Geometry: see drawing. Coordinates: mm, zero at the bounding-box minimum. A direction names the side the tool comes from. Give positions to 0.01 mm unless a question says otherwise; leave off trailing zeros. Write each loop counter-clockwise with the first axis right and the second up, starting at its lowest first coordinate (ties: lowest second). Pieces come first, ordered by that corner, then holes. Notation, with made-up numbers: (6, 65) - (22, 65) arc R25 ccw to (22, 79) - close; hole circle Ø3 at (-11, 9.5). An arc over 180 degrees is marked (long way). One line per question, with ' | ' between items. Start each with the question number.
(1) Ray query, line 1 (Y direction, x = 38, z = 48); line 2 (Y direction, x = 4, z = 13.5); line 3 (X direction, y = 17.5, z = 32). Return the intervals inside material, ascending. Write a range as [from, to].
(2) Section D-D, the plane y = 2. Return loops of the section in (x, z), plus the area to 3 significant figures.
(3) Section B-B, the plane x = 7.5. Return loops of the section in (y, z).
(4) Pin query (flat end, axial travel): pin 1 (5 mm diameter, centred on y = 22, z = 22.5, fed in from -X); pin 2 (1.5 mm diameter, centred on x = 38, y = 28, fed in from +Z). Return the tip coordinate at first contact, or that it passes through.
(5) Section A-A, the plane y = 23. Return loops of the section in (x, z), plus the area to 3 significant figures.
(6) Access query for the marked faces 5 and 6. Directions: +Z, -Z, +X, -X, +Y, -Y. A direction counts if a zero-diameter tool reaches every point of the face in a straight line with its end or side. Return the directions, or none.
(7) Draft query along Y for the marked faces 1, 2, 3 and 4. Return one class per face: +Y half, -Y half, draft (parallel to the pull), parting line (faces both ways), or undercut.
(8) Section C-C, the plane z = 37. Return loops of the section in (x, y), plus the area to 3 significant figures.
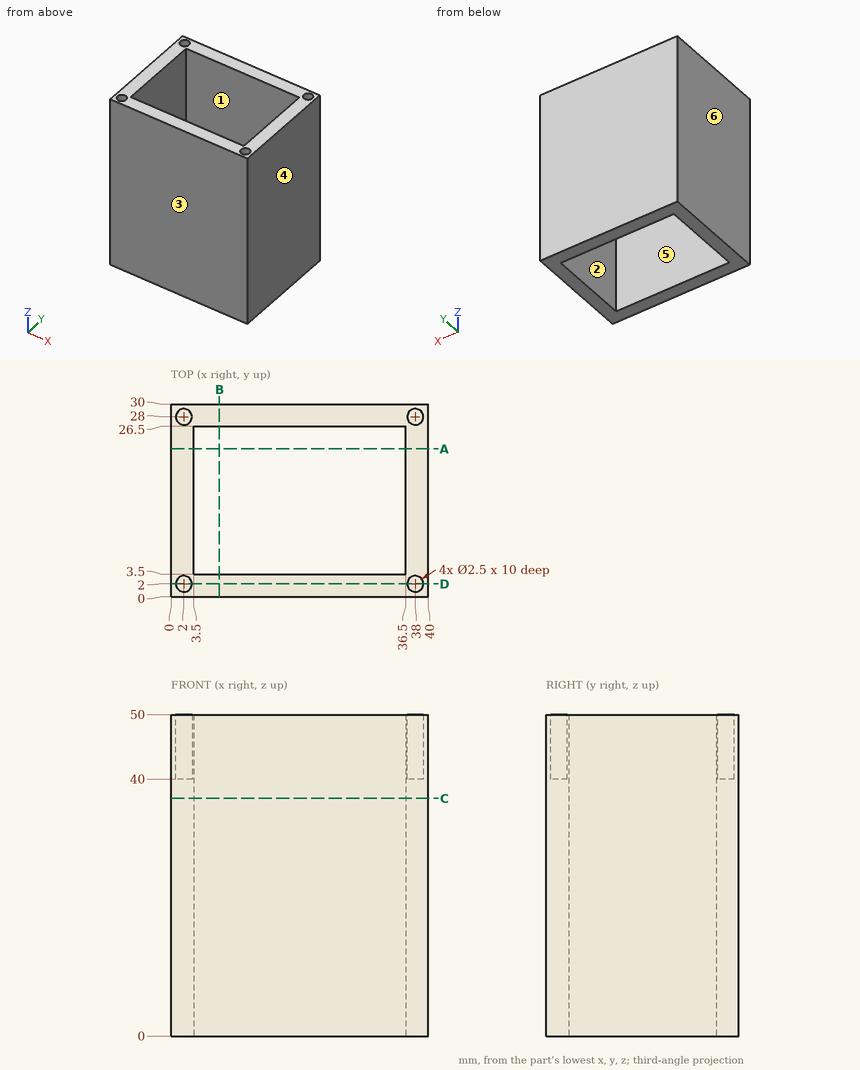
Check sheet entries:
1) line 1: [0, 0.75], [3.25, 26.75], [29.25, 30] | line 2: [0, 3.5], [26.5, 30] | line 3: [0, 3.5], [36.5, 40]
2) outline: (0, 0) - (40, 0) - (40, 50) - (39.25, 50) - (39.25, 40) - (36.75, 40) - (36.75, 50) - (3.25, 50) - (3.25, 40) - (0.75, 40) - (0.75, 50) - (0, 50) - close | area: 1,950 mm²
3) outline: (0, 0) - (3.5, 0) - (3.5, 50) - (0, 50) - close; (26.5, 0) - (30, 0) - (30, 50) - (26.5, 50) - close
4) pin 1: x = 0 | pin 2: z = 40
5) outline: (0, 0) - (3.5, 0) - (3.5, 50) - (0, 50) - close; (36.5, 0) - (40, 0) - (40, 50) - (36.5, 50) - close | area: 350 mm²
6) face 5: +Z, -Z | face 6: +Z, -Z, -X, +Y, -Y
7) face 1: undercut | face 2: undercut | face 3: -Y half | face 4: draft
8) outline: (0, 0) - (40, 0) - (40, 30) - (0, 30) - close; hole (3.5, 3.5) - (36.5, 3.5) - (36.5, 26.5) - (3.5, 26.5) - close | area: 441 mm²
